from build123d import *

# Parameters (mm, degrees)
F1_W     = 21.1428571429
F1_H     = 14.2857142857
F2_DEPTH = 1.1428571429
F3_W     = 21.1428571429
F3_H     = 14.2857142857
F4_DEPTH = 0.8571428571
F5_ANGLE = -97.1399716164
F7_DEPTH = 21.1428571429
F8_W     = 19.3768789759
F8_H     = 12.0920338668
F9_DEPTH = 0.2


with BuildPart() as f2:
    # F1 (on Top) → F2 (new body)
    with BuildSketch(Plane.XY):
        with Locations((10.5714285714, -7.1428571429)):
            Rectangle(F1_W, F1_H)
    extrude(amount=F2_DEPTH)



with BuildPart() as f4:
    # F3 (on face) → F4 (new body)
    with BuildSketch(Plane.XY.offset(1.1428571429)):
        with Locations((10.5714285714, -7.1428571429)):
            Rectangle(F3_W, F3_H)
    extrude(amount=F4_DEPTH)


with BuildPart() as f4_1:
    # F5: moved
    add(f4.part.rotate(Axis((10.5714285714, 0, 1.1428571429), (1, 0, 0)), F5_ANGLE))


with BuildPart() as f2_1:
    add(f2.part)

    add(f4_1.part)  # F7 merges F4
    # F6 (on face) → F7 (join, through all)
    with BuildSketch(Plane(origin=(0, 0, 0), x_dir=(0, -1, 0), z_dir=(-1, 0, 0))):
        Polygon((-0.850496115, 1.0363196571), (0, 0), (0, 1.1428571429), align=None)
    extrude(amount=-F7_DEPTH)

    # F8 (on face) → F9 (cut)
    with BuildSketch(Plane(origin=(0, -0.1409484498, 0.0176559225), x_dir=(1, 0, 0), z_dir=(0, -0.9922454675, 0.1242937334))):
        with Locations((10.5714288657, 8.1697662827)):
            Rectangle(F8_W, F8_H)
    extrude(amount=-F9_DEPTH, mode=Mode.SUBTRACT)


solid = f2_1.part
The listing builds one solid part. Answer for the finished solid, in the listing's coordinates (mm). A direction names the side the tool comes from. Round coordinates to 2 decimals unless told otherwise and drop trailing zeros. Write each loop counter-clockwise with the first axis right and the second up, starting at its lowest first coordinate (ties: lowest second). Pieces come first, ordered by that corner, then holes. Notation, with made-up numbers: M 9.25,85.5 L 66.25,85.5 A24 cw 66.25,108.5 Z; hole C 82.25,-40 d9. An arc over 180 degrees is marked long. Write each question's results on one line, items separated by ' | '. Start each with the question number.
(1) Find the intervals of material crossed by line 1 (Z direction, x = 9.25, y = -11.75); line 2 (Y direction, x = 12.5, z = 8.25); line 3 (Y direction, x = 4.25, z = 5), in increasing order.
(2) The part is cut by section C-C, the plane y = -9.75. Write down the section's boundary in (x, z).
(3) For faces 5 (the flat face through (10, -7, 1.143)), 6 (the flat face through (10.423, 1.726, 8.025)), determine the directions among +Z, -Z, +X, -X, +Y, -Y from which every point of the face is accessible in a straight line to the end or side of a thin tool.
(4) Each of these flat-tipped pins is pushed along its axis until it touches: P1, Ø2, axis at x = 11, z = 7.5, coming from the -Y side; P2, Ø4.5, axis at x = 14, y = -10.5, coming from the +Z side; P3, Ø1, axis at x = 18.5, z = 2.5, coming from the -Y side. Where does it stop, or does it pass through?
(5) The part is cut by section A-A, the plane x = 17.75. Write down the section's boundary in (y, z).
(6) Determine the mould class of faces 1 (the flat face through (10.423, 0.431, 0.525)), 2 (the flat face through (10.436, 1.083, 8.183)), 3 (the flat face through (0, -3.3, 0.9)), 4 (the flat face through (21.143, -3.3, 0.9)) for opening direction X: +X half, -X half, draft (parallel to the pull), parting line (faces both ways), or undercut.
(7) The part is cut by section B-B, the plane z = 13.75. Write down the section's boundary in (x, y), and give its area (3 significant figures).
Worked answers:
1) line 1: z = 0 to 1.14 | line 2: y = 1.09 to 1.75 | line 3: y = 0.68 to 1.35
2) outline: M 0,0 L 21.14,0 L 21.14,1.14 L 0,1.14 Z
3) face 5: +Z, +X, -X, -Y | face 6: -Z, +X, -X, +Y
4) P1: stops at y = 0.87 | P2: stops at z = 1.14 | P3: stops at y = 0.11
5) outline: M -14.29,0 L 0,0 L 0.85,1.04 L 2.63,15.21 L 1.78,15.32 L 1.63,14.12 L 1.82,14.1 L 0.32,2.1 L 0.12,2.12 L 0,1.14 L -14.29,1.14 Z
6) face 1: draft | face 2: undercut | face 3: -X half | face 4: +X half
7) outline: M 0,1.58 L 0.88,1.58 L 0.88,1.78 L 20.26,1.78 L 20.26,1.58 L 21.14,1.58 L 21.14,2.44 L 0,2.44 Z | area: 14.4 mm²
